Design review of the part built by this model. Coordinates are the model's own, in mm. A direction names the side the tool comes from. Coordinates: 2 decimals unless noted, no trailing zeros. Loops run counter-clockwise (first coordinate to the right, second up) from the corner with the lowest first, then second, coordinate; pieces in that order, holes last. Notation, with made-up numbers: M 73.25,48 L 118.25,48 A18 cw 118.25,62 Z; hole C -35.5,0.5 d7. An arc over 180 degrees is marked long. Put each result on its own line as item: value. Start each with the question number.
(1) Take a section at B-B, the plane x = -11.5. Give the boundary of the cut face in (y, z), then the cut area to 3 significant figures.
(2) Clearance check with a flat-ended pin moving along its axis: pin 1 (1.4 mm diameter, centred on x = 8, z = -24.5, fed in from +Y). State where the tip first meets the part, or that it passes through.
(3) For probe 1 along Z at (x, y) = (-23.5, 2.5); probe 2 along X at (y, z) = (3.35, -20); probe 3 along Y at (x, z) = (0, 12), list the stretches that pass through material, from the lowest coordinate up. Write a range as [from, to].
(4) Take a section at A-A, the plane y = 2.65. Give the boundary of the cut face in (x, z).
(5) For faces 5 (the flat face through (0, 2, 26.2)), 6 (the flat face through (0, 1.5, 0)), 7 (the flat face through (30.25, 2, 0)), list the 3-axis set-ups (+Z, -Z, +X, -X, +Y, -Y) from which the entire face can be reached by the end or side of a thin tool; tool diameter is ignored.
(6) The part is to be moulded in two halves that separate along Z. For faces 1 (the flat face through (0, 2, -22.15)), 2 (the flat face through (0, 1.5, 25)), 3 (the flat face through (0, 3.5, 27)), 4 (the flat face through (0, 2, -27.5)), say which applies: +Z half, -Z half, draft (parallel to the pull), parting line (faces both ways), or undercut.
(7) Take a section at C-C, the plane z = -5.5. Give the boundary of the cut face in (x, y), then the cut area to 4 significant figures.
```python
from build123d import *

# Parameters (mm, degrees)
SKETCH1_W           = 60.5
SKETCH1_H           = 55
BOSS_EXTRUDE1_DEPTH = 1.5
SKETCH2_W           = 60.5
SKETCH2_H           = 46.8
SKETCH2_W_2         = 58
SKETCH2_H_2         = 44.3
BOSS_EXTRUDE2_DEPTH = 2
SKETCH3_W           = 60.5
SKETCH3_H           = 1.3
BOSS_EXTRUDE3_DEPTH = 2


with BuildPart() as part:
    # Sketch1 → Boss-Extrude1 (new body)
    with BuildSketch(Plane(origin=(0, 0, 0), x_dir=(1, 0, 0), z_dir=(0, 1, 0))):
        Rectangle(SKETCH1_W, SKETCH1_H)
    extrude(amount=BOSS_EXTRUDE1_DEPTH)

    # Sketch2 → Boss-Extrude2 (add)
    with BuildSketch(Plane(origin=(0, 1.5, 0), x_dir=(1, 0, 0), z_dir=(0, 1, 0))):
        Rectangle(SKETCH2_W, SKETCH2_H)
        Rectangle(SKETCH2_W_2, SKETCH2_H_2, mode=Mode.SUBTRACT)
    extrude(amount=BOSS_EXTRUDE2_DEPTH)

    # Sketch3 → Boss-Extrude3 (add)
    with BuildSketch(Plane(origin=(0, 1.5, 0), x_dir=(1, 0, 0), z_dir=(0, 1, 0))):
        with Locations((0, 26.85)):
            Rectangle(SKETCH3_W, SKETCH3_H)
        with Locations((0, -26.85)):
            Rectangle(SKETCH3_W, SKETCH3_H)
    extrude(amount=BOSS_EXTRUDE3_DEPTH)


solid = part.part
```
Computed values:
1. outline: M 0,-27.5 L 3.5,-27.5 L 3.5,-26.2 L 1.5,-26.2 L 1.5,-23.4 L 3.5,-23.4 L 3.5,-22.15 L 1.5,-22.15 L 1.5,22.15 L 3.5,22.15 L 3.5,23.4 L 1.5,23.4 L 1.5,26.2 L 3.5,26.2 L 3.5,27.5 L 0,27.5 Z
1. area: 92.7 mm^2
2. pin 1: stops at y = 1.5
3. probe 1: z = [-27.5, -26.2], [-23.4, -22.15], [22.15, 23.4], [26.2, 27.5]
3. probe 2: x = [-30.25, -29], [29, 30.25]
3. probe 3: y = [0, 1.5]
4. outline: M -30.25,-27.5 L 30.25,-27.5 L 30.25,-26.2 L -30.25,-26.2 Z; M -30.25,-23.4 L 30.25,-23.4 L 30.25,23.4 L -30.25,23.4 Z; M -30.25,26.2 L 30.25,26.2 L 30.25,27.5 L -30.25,27.5 Z; hole M -29,-22.15 L 29,-22.15 L 29,22.15 L -29,22.15 Z
5. face 5: +X, -X, +Y
5. face 6: +Y
5. face 7: +Z, -Z, +X, +Y, -Y
6. face 1: undercut
6. face 2: undercut
6. face 3: draft
6. face 4: -Z half
7. outline: M -30.25,0 L 30.25,0 L 30.25,3.5 L 29,3.5 L 29,1.5 L -29,1.5 L -29,3.5 L -30.25,3.5 Z
7. area: 95.75 mm^2
